Check sheet for the modelled part. Datum: model origin and axes. Units: mm. A direction names the side the tool comes from. Round coordinates to 2 decimals unless told otherwise and drop trailing zeros. Loops run counter-clockwise (first coordinate to the right, second up) from the corner with the lowest first, then second, coordinate; pieces in that order, holes last. Notation, with made-up numbers: (-21, 21.5) -> (29, 21.5) arc R33 ccw to (29, 59.5) -> close; hole circle Ø4 at (25, -18). An arc over 180 degrees is marked (long way). Return JSON: item names as keys, results as strings.
from build123d import *

# Parameters (mm, degrees)
SKETCH1_W                                      = 45
SKETCH1_H                                      = 73
SKETCH1_R                                      = 20.25
BOSS_EXTRUDE1_DEPTH                            = 5
CHAMFER1_SIZE                                  = 4
SKETCH2_W                                      = 45
SKETCH2_H                                      = 17
BOSS_EXTRUDE2_DEPTH                            = 32.5
CBORE_SLOT_FOR_M6_HEX_SOCKET_HEAD_CAP_SC_DEPTH = 17
CBORE_START                                    = 10.5
CBORE_SLOT_FOR_M6_HEX_SOCKET_HEAD_CA_3_DEPTH   = 6.5
BOSS_EXTRUDE3_DEPTH                            = 2.5
FILLET1_R                                      = 3
FILLET1_OF_MIRROR1_R                           = 3


# Read off the part's stored shape, not the designer's step: CBORE SLOT for M6 Hex Socket Head Cap Screw1
with BuildPart() as part:
    # Sketch1 → Boss-Extrude1 (new body)
    with BuildSketch(Plane(origin=(0, 0, 0), x_dir=(0, 0, -1), z_dir=(1, 0, 0))):
        with Locations((0, 36.5)):
            Rectangle(SKETCH1_W, SKETCH1_H)
        with Locations((0, 47.5)):
            Circle(SKETCH1_R, mode=Mode.SUBTRACT)
    extrude(amount=BOSS_EXTRUDE1_DEPTH)

    # Chamfer1
    chamfer1_edges = [part.edges().sort_by_distance(p)[0] for p in [
        (2.5, 73, 22.5),
        (2.5, 73, -22.5),
    ]]
    chamfer(chamfer1_edges, length=CHAMFER1_SIZE)

    # Sketch2 → Boss-Extrude2 (add)
    with BuildSketch(Plane.ZY):
        with Locations((0, 8.5)):
            Rectangle(SKETCH2_W, SKETCH2_H)
    extrude(amount=BOSS_EXTRUDE2_DEPTH)

    # CBORE SLOT for M6 Hex Socket Head Ca 2 → CBORE SLOT for M6 Hex Socket Head Cap Screw1 (cut)
    with BuildSketch(Plane(origin=(0, 0, 0), x_dir=(1, 0, 0), z_dir=(0, 1, 0))):
        with BuildLine():
            Line((-24.2, -15.8), (-5.8, -15.8))
            ThreePointArc((-5.8, -15.8), (-2.5, -12.5), (-5.8, -9.2))
            Line((-5.8, -9.2), (-24.2, -9.2))
            ThreePointArc((-24.2, -9.2), (-27.5, -12.5), (-24.2, -15.8))
        make_face()
        with BuildLine():
            Line((-24.2, 9.2), (-5.8, 9.2))
            ThreePointArc((-5.8, 9.2), (-2.5, 12.5), (-5.8, 15.8))
            Line((-5.8, 15.8), (-24.2, 15.8))
            ThreePointArc((-24.2, 15.8), (-27.5, 12.5), (-24.2, 9.2))
        make_face()
    extrude(amount=CBORE_SLOT_FOR_M6_HEX_SOCKET_HEAD_CAP_SC_DEPTH, mode=Mode.SUBTRACT)

    # CBORE SLOT for M6 Hex Socket Head Ca 3 o → CBORE SLOT for M6 Hex Socket Head Ca 3 (cut)
    # profile 1 of 2: a face of its own
    with BuildSketch(Plane(origin=(0, 0, 0), x_dir=(1, 0, 0), z_dir=(0, 1, 0)).offset(CBORE_START)):
        with BuildLine():
            Line((-24.2, -18), (-5.8, -18))
            ThreePointArc((-5.8, -18), (-0.3, -12.5), (-5.8, -7))
            Line((-5.8, -7), (-24.2, -7))
            ThreePointArc((-24.2, -7), (-29.7, -12.5), (-24.2, -18))
        make_face()
        with BuildLine():
            ThreePointArc((-5.8, -9.2), (-2.5, -12.5), (-5.8, -15.8))
            Line((-5.8, -15.8), (-24.2, -15.8))
            ThreePointArc((-24.2, -15.8), (-27.5, -12.5), (-24.2, -9.2))
            Line((-24.2, -9.2), (-5.8, -9.2))
        make_face(mode=Mode.SUBTRACT)
    # profile 2 of 2: a face of its own
    with BuildSketch(Plane(origin=(0, 0, 0), x_dir=(1, 0, 0), z_dir=(0, 1, 0)).offset(CBORE_START)):
        with BuildLine():
            Line((-24.2, 7), (-5.8, 7))
            ThreePointArc((-5.8, 7), (-0.3, 12.5), (-5.8, 18))
            Line((-5.8, 18), (-24.2, 18))
            ThreePointArc((-24.2, 18), (-29.7, 12.5), (-24.2, 7))
        make_face()
        with BuildLine():
            ThreePointArc((-5.8, 15.8), (-2.5, 12.5), (-5.8, 9.2))
            Line((-5.8, 9.2), (-24.2, 9.2))
            ThreePointArc((-24.2, 9.2), (-27.5, 12.5), (-24.2, 15.8))
            Line((-24.2, 15.8), (-5.8, 15.8))
        make_face(mode=Mode.SUBTRACT)
    extrude(amount=CBORE_SLOT_FOR_M6_HEX_SOCKET_HEAD_CA_3_DEPTH, mode=Mode.SUBTRACT)

    # Sketch5 → Boss-Extrude3 (add)
    with BuildSketch(Plane.XY.offset(22.5)):
        Polygon((0, 37), (-32.5, 17), (0, 17), align=None)
    boss_extrude3 = extrude(amount=-BOSS_EXTRUDE3_DEPTH)

    # Fillet1
    # the kernel refuses this fillet: 3 mm, written as the material it adds along each edge
    with BuildSketch(Plane(origin=(0, 9.5, 20), x_dir=(0, 0, -1), z_dir=(0, 1, 0))) as fillet1_piece_1_section:
        with BuildLine():
            CenterArc((FILLET1_R, FILLET1_R), FILLET1_R, 180, 90)
            Line((0, FILLET1_R), (0, 0))
            Line((0, 0), (FILLET1_R, 0))
        make_face()
    fillet1_piece_1 = extrude(amount=35, mode=Mode.PRIVATE)
    fillet1_piece_1 = split(fillet1_piece_1, bisect_by=Plane(origin=(-11.093486365, 30.17323916, 19.320814657), z_dir=(0.5240974256643348, -0.8516583167045438, 0)), keep=Keep.TOP, mode=Mode.PRIVATE)
    fillet1_piece_1 = fillet1_piece_1 - Plane(origin=(-0.679185343, 47.5, 0), x_dir=(0, 0, -1), z_dir=(-1, 0, 0)) * Cylinder(20.25, 83, mode=Mode.PRIVATE)
    add(fillet1_piece_1)

    # Mirror1: Boss-Extrude3 across plane
    add(boss_extrude3.mirror(Plane.XY))

    # Fillet1 of Mirror1
    # the kernel refuses this fillet: 3 mm, written as the material it adds along each edge
    with BuildSketch(Plane(origin=(0, 9.5, -20), x_dir=(0, 0, 1), z_dir=(0, 1, 0))) as fillet1_of_mirror1_piece_1_section:
        with BuildLine():
            CenterArc((FILLET1_OF_MIRROR1_R, -FILLET1_OF_MIRROR1_R), FILLET1_OF_MIRROR1_R, 90, 90)
            Line((0, -FILLET1_OF_MIRROR1_R), (0, 0))
            Line((0, 0), (FILLET1_OF_MIRROR1_R, 0))
        make_face()
    fillet1_of_mirror1_piece_1 = extrude(amount=35, mode=Mode.PRIVATE)
    fillet1_of_mirror1_piece_1 = fillet1_of_mirror1_piece_1 - Plane(origin=(-0.679185343, 47.5, 0), x_dir=(0, 0, -1), z_dir=(-1, 0, 0)) * Cylinder(20.25, 83, mode=Mode.PRIVATE)
    fillet1_of_mirror1_piece_1 = split(fillet1_of_mirror1_piece_1, bisect_by=Plane(origin=(-11.093486365, 30.17323916, -19.320814657), z_dir=(0.5240974256643348, -0.8516583167045438, 0)), keep=Keep.TOP, mode=Mode.PRIVATE)
    add(fillet1_of_mirror1_piece_1)


solid = part.part
Q1. Section check A-A (z = 0). Record the boundary of the cut face in (x, y).
Results list:
{"outline": "(-32.5, 0) -> (5, 0) -> (5, 27.25) -> (0, 27.25) -> (0, 17) -> (-32.5, 17) -> close; (0, 67.75) -> (5, 67.75) -> (5, 73) -> (0, 73) -> close"}
Q2. Section check D-D (z = -12). Record the boundary of the cut face in (x, y), then the cut area to 3 significant figures.
Results list:
{"outline": "(-32.5, 0) -> (-27.46, 0) -> (-27.46, 10.5) -> (-29.68, 10.5) -> (-29.68, 17) -> (-32.5, 17) -> close; (-2.54, 0) -> (5, 0) -> (5, 31.19) -> (0, 31.19) -> (0, 17) -> (-0.32, 17) -> (-0.32, 10.5) -> (-2.54, 10.5) -> close; (0, 63.81) -> (5, 63.81) -> (5, 73) -> (0, 73) -> close", "area": "302 mm^2"}
Q3. Section check B-B (y = 47.5). Record the boundary of the cut face in (x, z).
Results list:
{"outline": "(0, -22.5) -> (5, -22.5) -> (5, -20.25) -> (0, -20.25) -> close; (0, 20.25) -> (5, 20.25) -> (5, 22.5) -> (0, 22.5) -> close"}
Q4. Draft check along Z on faces 4 (the flat face through (2, 73, 0)), 5 (the flat face through (-11, 22, 20)), 6 (the flat face through (2.5, 71, -20.5)). Enter one of: released by +Z, released by -Z, zero draft, split by the parting line, or undercut.
Results list:
{"face 4": "zero draft", "face 5": "undercut", "face 6": "released by -Z"}
Q5. Section check C-C (x = -18). Record the boundary of the cut face in (y, z).
Results list:
{"outline": "(0, -22.5) -> (25.92, -22.5) -> (25.92, -20) -> (17, -20) -> (17, -18) -> (10.5, -18) -> (10.5, -15.8) -> (0, -15.8) -> close; (0, -9.2) -> (10.5, -9.2) -> (10.5, -7) -> (17, -7) -> (17, 7) -> (10.5, 7) -> (10.5, 9.2) -> (0, 9.2) -> close; (0, 15.8) -> (10.5, 15.8) -> (10.5, 18) -> (17, 18) -> (17, 20) -> (25.92, 20) -> (25.92, 22.5) -> (0, 22.5) -> close"}
Q6. Go/stop test with flat-tipped pins: pin 1 (18 mm diameter, centred on y = 51.5, z = 8.5, fed in from -X); pin 2 (1.5 mm diameter, centred on x = -12, z = -16.5, fed in from -Y); pin 3 (9 mm diameter, centred on x = -19, z = 13, fed in from +Y); pin 4 (10 mm diameter, centred on y = 23.5, z = 10.5, fed in from -X). Record where each tip stops, or that it passes through.
Results list:
{"pin 1": "through", "pin 2": "y = 0", "pin 3": "y = 10.5", "pin 4": "x = 0"}
Q7. Material ranges on line 1 (Y direction, x = 1.05, z = 0); line 2 (Z direction, x = 3.3, y = 47.5); line 3 (Z direction, x = -1, y = 15), recorded low to high.
Results list:
{"line 1": "0 to 27.25, 67.75 to 73", "line 2": "-22.5 to -20.25, 20.25 to 22.5", "line 3": "-22.5 to -15.19, -9.81 to 9.81, 15.19 to 22.5"}
Q8. Tool access check on faces 1 (the flat face through (-15, 14, -18)), 2 (the flat face through (-11, 22, -20)), 3 (the flat face through (-15, 5, 9.2)). Record the directions out of +Z, -Z, +X, -X, +Y, -Y that give a thin tool (end or side, any length) a straight path to the whole face; none if there is none.
Results list:
{"face 1": "+Y", "face 2": "-X, +Y", "face 3": "+Y, -Y"}
